from build123d import *

# Parameters (mm, degrees)
BOSS_EXTRUDE1_DEPTH = 11
SHELL1_T            = -2
FILLET1_R           = 1


with BuildPart() as part:
    # Sketch1 → Boss-Extrude1 (new body)
    with BuildSketch(Plane(origin=(0, 0, 0), x_dir=(1, 0, 0), z_dir=(0, 1, 0))):
        with BuildLine():
            Line((0, 0), (0, 30))
            Line((0, 30), (15.92, 30))
            ThreePointArc((15.92, 30), (13.000920011, 15), (15.92, 0))
            Line((15.92, 0), (0, 0))
        make_face()
    extrude(amount=BOSS_EXTRUDE1_DEPTH)

    # Shell1
    shell1_openings = [part.faces().sort_by_distance(p)[0] for p in [
        (7.00647131, 0, -15),
        (13.000920011, 5.5, -15),
    ]]
    offset(amount=SHELL1_T, openings=shell1_openings, kind=Kind.INTERSECTION)

    # Fillet1
    fillet1_edges = [part.edges().sort_by_distance(p)[0] for p in [
        (7.96, 11, -30),
        (0, 11, -15),
        (7.96, 11, 0),
        (0, 5.5, 0),
        (0, 5.5, -30),
        (13.000920011, 11, -15),
    ]]
    fillet(fillet1_edges, radius=FILLET1_R)


solid = part.part
Here's how the part is built. I have some questions about the finished solid (model axes, mm). A direction names the side the tool comes from. Coordinates: 2 decimals unless noted, no trailing zeros. Order: outer loops, then holes, each group sorted by start corner. A loop starts at its lowest first (then second) coordinate and runs counter-clockwise, first axis right, second up. Notation, with made-up numbers: (-16.75, 53) - (7.25, 53) arc R31 ccw to (7.25, 77) - close; hole circle Ø8 at (-38, 59.5). An arc over 180 degrees is marked (long way). Use CSV: the item, a comma, the result in double quotes. Start each with the question number.
1. I'm going to push flat-ended pins straight in: pin 1 (4.5 mm diameter, centred on y = 3, z = -14.5, fed in from +X); pin 2 (1.5 mm diameter, centred on x = 9.5, z = -11, fed in from -Y). Where does each tip first touch, or does it pass through?
2. Suppose I cut it at B-B on y = 8. List the corners of the cut face in (x, z) for me, then the cut area to 3 significant figures.
3. Suppose I cut it at A-A on x = 5.75. List the corners of the cut face in (y, z) for me, then the cut area to 3 significant figures.
4. If we mould it in two halves opening along Z, with no side actions, what happens to faces 1 (the face through (9, 9, -15)), 2 (the face through (1.5, 0, -15.1)), 3 (the face through (8.564, 10.699, -29.715))? For each: +Z half, -Z half, draft (parallel to the pull), parting line (faces both ways), or undercut.
5. For faces 4 (the face through (8, 4, -28)), 5 (the face through (8.356, 10.699, -0.285)), which set-ups out of +Z, -Z, +X, -X, +Y, -Y let a thin tool reach every point of the face, with its end or its side?
6. Please list where these lines run through material, in increasing order: line 1 (Z direction, x = 6.25, y = 7); line 2 (Y direction, x = 7, z = -7.5); line 3 (X direction, y = 1.75, z = -14). Write a range as from..to.
Output:
1,pin 1,"stops at x = 2"
1,pin 2,"stops at y = 9"
2,outline,"(0, -29) arc R1 ccw to (1, -30) - (15.92, -30) arc R40 cw to (15.17, -28) - (2, -28) - (2, -2) - (15.17, -2) arc R40 cw to (15.92, 0) - (1, 0) arc R1 ccw to (0, -1) - close"
2,area,"114 mm2"
3,outline,"(0, -30) - (10, -30) arc R1 ccw to (11, -29) - (11, -1) arc R1 ccw to (10, 0) - (0, 0) - (0, -2) - (9, -2) - (9, -28) - (0, -28) - close"
3,area,"95.6 mm2"
4,face 1,"undercut"
4,face 2,"draft"
4,face 3,"-Z half"
5,face 4,"+X, -Y"
5,face 5,"+Z, +X, -X, +Y"
6,line 1,"z = -30..-28, -2..0"
6,line 2,"y = 9..11"
6,line 3,"x = 0..2"
